Can you work these out from the model? Positions are in its coordinate system, mm. A direction names the side the tool comes from. Round coordinates to 2 decimals unless told otherwise and drop trailing zeros. Loops run counter-clockwise (first coordinate to the right, second up) from the corner with the lowest first, then second, coordinate; pieces in that order, holes last. Notation, with made-up numbers: M -18,3.5 L -2,3.5 A22 cw -2,37.5 Z; hole C 77,-27.5 d3. An arc over 180 degrees is marked long. Return JSON: item names as keys, results as strings.
```python
from build123d import *

# Parameters (mm, degrees)
F0_R     = 44.863573
F1_DEPTH = 63.5
F2_R     = 38.515034
F3_DEPTH = 25.4
F4_R     = 6.510435
F5_DEPTH = 63.5


with BuildPart() as f1:
    # F0 (on Front) → F1 (new body)
    with BuildSketch(Plane.XZ):
        Circle(F0_R)
    extrude(amount=F1_DEPTH)

    # F2 (on face) → F3 (cut)
    with BuildSketch(Plane(origin=(0, 0, 0), x_dir=(-1, 0, 0), z_dir=(0, 1, 0))):
        Circle(F2_R)
    extrude(amount=-F3_DEPTH, mode=Mode.SUBTRACT)

    # F4 (on face) → F5 (cut)
    with BuildSketch(Plane.XZ.offset(63.5)):
        Circle(F4_R)
    extrude(amount=-F5_DEPTH, mode=Mode.SUBTRACT)


solid = f1.part
```
Q1. Suppose I cut it at C-C, the plane y = -54.5. Please give me the cut outline in (x, z).
Results:
{"outline": "C 0,0 d89.73; hole C 0,0 d13.02"}
Q2. Suppose I cut it at B-B, the plane x = 0. Please give me the cut outline in (y, z), plus the area to 3 significant figures.
Results:
{"outline": "M -63.5,-44.86 L 0,-44.86 L 0,-38.52 L -25.4,-38.52 L -25.4,-6.51 L -63.5,-6.51 Z; M -63.5,6.51 L -25.4,6.51 L -25.4,38.52 L 0,38.52 L 0,44.86 L -63.5,44.86 Z", "area": "3,250 mm2"}
Q3. I'm going to push flat-ended pins straight in: pin 1 Ø2 at (x, y) = (-34, -37.5) entering from -Z; pin 2 Ø4 at (x, y) = (-18, -49) entering from +Z; pin 3 Ø4 at (x, y) = (-11, -6.5) entering from +Z; pin 4 Ø8 at (x, z) = (0, 0) entering from +Y. Where does each tip first touch, or does it pass through?
Results:
{"pin 1": "stops at z = -30.39", "pin 2": "stops at z = 41.91", "pin 3": "stops at z = 43.95", "pin 4": "passes through"}
Q4. On a 3-axis mill with a long thin cutter (end or side, diameter ignored), from which of +Z, -Z, +X, -X, +Y, -Y can I reach the whole of each face in a straight line? I mean faces 1 (the flat face through (-1, -63.5, -9)), 2 (the cylindrical face through (8.35, -12.52, -37.6)). Say none if no direction works.
Results:
{"face 1": "+Z, -Z, +X, -X, -Y", "face 2": "+Y"}
Q5. Thinking about a two-plate mould opening in Z: for faces 3 (the cylindrical face through (6.014, -44.717, -2.494)), 4 (the flat face through (19.7, 0, 33.4)), 5 (the cylindrical face through (24.12, -31.31, 37.83)), which applies, pulls with the +Z half, pulls with the -Z half, needs draft (parallel to the pull), parting line crosses it, or undercut?
Results:
{"face 3": "undercut", "face 4": "needs draft", "face 5": "parting line crosses it"}
Q6. Suppose I cut it at A-A, the plane z = 0. Please give me the cut outline in (x, y).
Results:
{"outline": "M -44.86,-63.5 L -6.51,-63.5 L -6.51,-25.4 L -38.52,-25.4 L -38.52,0 L -44.86,0 Z; M 6.51,-63.5 L 44.86,-63.5 L 44.86,0 L 38.52,0 L 38.52,-25.4 L 6.51,-25.4 Z"}
Q7. If I drill on line 1 along Z through (x, y) = (0, -11.25); line 2 along Z through (x, y) = (0, -32); line 3 along X through (y, z) = (-16, -1), over which ranges is the centre line in solid material (lowest first)?
Results:
{"line 1": "z = -44.86 to -38.52, 38.52 to 44.86", "line 2": "z = -44.86 to -6.51, 6.51 to 44.86", "line 3": "x = -44.85 to -38.5, 38.5 to 44.85"}
Q8. Suppose I cut it at D-D, the plane z = -30.5. Please give me the cut outline in (x, y).
Results:
{"outline": "M -32.9,-63.5 L 32.9,-63.5 L 32.9,0 L 23.52,0 L 23.52,-25.4 L -23.52,-25.4 L -23.52,0 L -32.9,0 Z"}
